from build123d import *

# Parameters (mm, degrees)
SKETCH_1_R          = 1.5
SKETCH_1_R_2        = 5
EXTRUDE_1_DEPTH     = 5
SKETCH_2_R          = 6.5
CUT_EXTRUDE_1_DEPTH = 3
FILLET_1_R          = 4


with BuildPart() as part:
    # Эскиз1 → Бобышка-Вытянуть1 (new body)
    with BuildSketch(Plane(origin=(0, -185.809804521, 0), x_dir=(1, 0, 0), z_dir=(0, 1, 0))):
        with BuildLine():
            Line((-450.111062941, 89.302859511), (-450.111062941, 76.302859511))
            Line((-450.111062941, 76.302859511), (-476.111062941, 76.302859511))
            Line((-476.111062941, 76.302859511), (-491.742757589, 81.748272926))
            ThreePointArc((-491.742757589, 81.748272926), (-497.110912638, 89.302859511), (-491.742757589, 96.857446095))
            Line((-491.742757589, 96.857446095), (-476.111062941, 102.302859511))
            Line((-476.111062941, 102.302859511), (-450.111062941, 102.302859511))
            Line((-450.111062941, 102.302859511), (-450.111062941, 89.302859511))
        make_face()
        with Locations(Location((-470.811062941, 96.102859511, 0), (0, 0, 270))):
            Circle(SKETCH_1_R, mode=Mode.SUBTRACT)
        with Locations(Location((-455.411062941, 96.102859511, 0), (0, 0, 270))):
            Circle(SKETCH_1_R, mode=Mode.SUBTRACT)
        with Locations(Location((-455.411062941, 82.502859511, 0), (0, 0, 270))):
            Circle(SKETCH_1_R, mode=Mode.SUBTRACT)
        with Locations(Location((-470.811062941, 82.502859511, 0), (0, 0, 270))):
            Circle(SKETCH_1_R, mode=Mode.SUBTRACT)
        with Locations(Location((-463.111062941, 89.302859511, 0), (0, 0, 270))):
            Circle(SKETCH_1_R_2, mode=Mode.SUBTRACT)
        with Locations(Location((-489.111062941, 89.302859511, 0), (0, 0, 270))):
            Circle(SKETCH_1_R_2, mode=Mode.SUBTRACT)
    extrude(amount=EXTRUDE_1_DEPTH)

    # Эскиз2 → Вырез-Вытянуть1 (cut)
    with BuildSketch(Plane(origin=(0, -180.809804521, 0), x_dir=(1, 0, 0), z_dir=(0, 1, 0))):
        with Locations(Location((-463.111062941, 89.302859511, 0), (0, 0, 270))):
            Circle(SKETCH_2_R)
        with Locations(Location((-489.111062941, 89.302859511, 0), (0, 0, 270))):
            Circle(SKETCH_2_R)
    extrude(amount=-CUT_EXTRUDE_1_DEPTH, mode=Mode.SUBTRACT)

    # Скругление1
    fillet_1_edges = [part.edges().sort_by_distance(p)[0] for p in [
        (-476.111062941, -183.309804521, -102.302859511),
        (-450.111062941, -183.309804521, -102.302859511),
        (-450.111062941, -183.309804521, -76.302859511),
        (-476.111062941, -183.309804521, -76.302859511),
    ]]
    fillet(fillet_1_edges, radius=FILLET_1_R)


solid = part.part
Input: part model. Units: mm. Frame: model coordinates. A direction names the side the tool comes from. Give positions to 0.01 mm unless a question says otherwise; leave off trailing zeros. Order: outer loops, then holes, each group sorted by start corner. A loop starts at its lowest first (then second) coordinate and runs counter-clockwise, first axis right, second up.
Q1. Set-up query: faces 1 (the flat face through (-466, -183.81, -85)), 2 (the flat face through (-450.111, -183, -89)). Return all of +Z, -Z, +X, -X, +Y, -Y with unobstructed straight access to the full face (end or side cutting, diameter ignored); none if empty.
Checked values:
face 1: +Y
face 2: +Z, -Z, +X, +Y, -Y
Q2. Section C-C on y = -181.75. Output: boundary loops of the cut face in (x, z), and give its area (3 significant figures).
Checked values:
outline: (-491.74, -96.86) - (-476.75, -102.08) arc R4 ccw to (-475.43, -102.3) - (-454.11, -102.3) arc R4 ccw to (-450.11, -98.3) - (-450.11, -80.3) arc R4 ccw to (-454.11, -76.3) - (-475.43, -76.3) arc R4 ccw to (-476.75, -76.53) - (-491.74, -81.75) arc R8 ccw to start; hole circle Ø13 at (-489.11, -89.3); hole circle Ø3 at (-470.81, -96.1); hole circle Ø3 at (-470.81, -82.5); hole circle Ø13 at (-463.11, -89.3); hole circle Ø3 at (-455.41, -96.1); hole circle Ø3 at (-455.41, -82.5)
area: 756 mm2
Q3. Section B-B on x = -462. Output: boundary loops of the cut face in (y, z).
Checked values:
outline: (-185.81, -102.3) - (-180.81, -102.3) - (-180.81, -95.71) - (-183.81, -95.71) - (-183.81, -94.18) - (-185.81, -94.18) - close; (-185.81, -84.43) - (-183.81, -84.43) - (-183.81, -82.9) - (-180.81, -82.9) - (-180.81, -76.3) - (-185.81, -76.3) - close
Q4. Contact query for flat-ended pins moving along their axis: pin 1 Ø10.5 at (x, z) = (-491, -90) entering from +Y; pin 2 Ø10.5 at (x, z) = (-489.11, -89.3) entering from +Y; pin 3 Ø1.5 at (x, y) = (-484, -181.5) entering from -Z; pin 4 Ø1.5 at (x, y) = (-479, -182) entering from +Z. Output: stop coordinate, or through.
Checked values:
pin 1: stops at y = -180.81
pin 2: stops at y = -183.81
pin 3: stops at z = -99.82
pin 4: stops at z = -77.05
Q5. Ray query, probe 1 along X at (y, z) = (-183.3, -89); probe 2 along X at (y, z) = (-183.45, -91.5); probe 3 along Z at (x, y) = (-471, -181.95). Return the intervals inside material, ascending.
Checked values:
probe 1: x = -497.11 to -495.6, -482.62 to -469.6, -456.62 to -450.11
probe 2: x = -496.8 to -495.23, -482.99 to -469.23, -456.99 to -450.11
probe 3: z = -102.3 to -97.59, -94.61 to -83.99, -81.01 to -76.3
Q6. Section A-A on z = -96.25. Output: boundary loops of the cut face in (x, y), and give its area (3 significant figures).
Checked values:
outline: (-493.08, -185.81) - (-472.3, -185.81) - (-472.3, -180.81) - (-493.08, -180.81) - close; (-469.32, -185.81) - (-456.9, -185.81) - (-456.9, -180.81) - (-469.32, -180.81) - close; (-453.92, -185.81) - (-450.11, -185.81) - (-450.11, -180.81) - (-453.92, -180.81) - close
area: 185 mm2
Q7. Section D-D on z = -89.75. Output: boundary loops of the cut face in (x, y), and give its area (3 significant figures).
Checked values:
outline: (-497.1, -185.81) - (-494.09, -185.81) - (-494.09, -183.81) - (-495.6, -183.81) - (-495.6, -180.81) - (-497.1, -180.81) - close; (-484.13, -185.81) - (-468.09, -185.81) - (-468.09, -183.81) - (-469.6, -183.81) - (-469.6, -180.81) - (-482.63, -180.81) - (-482.63, -183.81) - (-484.13, -183.81) - close; (-458.13, -185.81) - (-450.11, -185.81) - (-450.11, -180.81) - (-456.63, -180.81) - (-456.63, -183.81) - (-458.13, -183.81) - close
area: 117 mm2
Q8. Draft query along Z for faces 3 (the cylindrical face through (-451.25, -183.27, -101.1)), 4 (the cylindrical face through (-453.924, -183.345, -96.298)), 5 (the cylindrical face through (-476.092, -183.275, -76.357)). Return one class per face: +Z half, -Z half, draft (parallel to the pull), parting line (faces both ways), or undercut.
Checked values:
face 3: -Z half
face 4: undercut
face 5: +Z half
